Check sheet for the modelled part. Datum: model origin and axes. Units: mm. A direction names the side the tool comes from. Coordinates: 2 decimals unless noted, no trailing zeros. Loops run counter-clockwise (first coordinate to the right, second up) from the corner with the lowest first, then second, coordinate; pieces in that order, holes last. Notation, with made-up numbers: (39, 9) - (83, 9) arc R20 cw to (83, 16) - close; hole circle Ø10 at (54.25, 68). An arc over 180 degrees is marked (long way). Use a Markdown table: item, result. Add a question column.
1) Sectioned sample at D-D, the plane z = 159. Enter the section's corners in (x, y).
2) Sectioned sample at A-A, the plane y = -52. Enter the section's corners in (x, z) (1 decimal).
3) Draft check along Z on faces 6 (the flat face through (4, 1, -15.875)), 7 (the flat face through (-377, 1, 619.125)), 8 (the flat face through (3, -63.343, 0)), 9 (the cylindrical face through (-161.17, -12, 297.62)). Enter one of: pulls with the +Z half, pulls with the -Z half, needs draft (parallel to the pull), parting line crosses it, or undercut.
4) Go/stop test with flat-tipped pins: P1, Ø8, axis at x = 13.5, y = -45, coming from the +Z side (3 decimals); P2, Ø1.5, axis at y = -2, z = 51.5, coming from the -X side; P3, Ø4, axis at y = 12.5, z = 183.5, coming from the -X side. Record where each tip stops, or that it passes through.
5) Sectioned sample at B-B, the plane z = 606. Enter the section's corners in (x, y).
6) Thickness scan on line 1 (Z direction, x = -551, y = 48.5) (3 decimals); line 2 (Z direction, x = -14, y = 47.5) (3 decimals); line 3 (X direction, y = -1, z = 445). Record the ranges inside material, lowest first.
7) Tool access check on faces 1 (the cylindrical face through (-554.43, 26.93, 681.74)), 2 (the flat face through (-384, 63.657, 603)), 3 (the cylindrical face through (-253.985, -1.239, 0.222)), 4 (the cylindrical face through (-127.015, 1.554, 603.472)), 5 (the cylindrical face through (219.83, -12, -96.36)). Record the directions out of +Z, -Z, +X, -X, +Y, -Y that give a thin tool (end or side, any length) a straight path to the whole face; none if there is none.
8) Sectioned sample at C-C, the plane x = -477. Enter the section's corners in (y, z) (3 decimals).
from build123d import *

# Parameters (mm, degrees)
SKETCH1_R           = 31.75
BOSS_EXTRUDE1_DEPTH = 15.875
SKETCH2_R           = 31.75
BOSS_EXTRUDE2_DEPTH = 571.5
BOSS_EXTRUDE3_START = -190.5
SKETCH4_R           = 31.75
BOSS_EXTRUDE3_DEPTH = 190.5
BOSS_EXTRUDE4_START = 31.75
BOSS_EXTRUDE4_DEPTH = 31.75
SKETCH7_R           = 31.75
BOSS_EXTRUDE5_DEPTH = 127


with BuildPart() as part:
    # Sketch1 → Boss-Extrude1 (new, symmetric)
    with BuildSketch(Plane.XY):
        with BuildLine():
            Line((-190.5, 63.657439452), (190.5, 63.657439452))
            ThreePointArc((190.5, 63.657439452), (254, 0.157439452), (190.5, -63.342560548))
            Line((190.5, -63.342560548), (-190.5, -63.342560548))
            ThreePointArc((-190.5, -63.342560548), (-254, 0.157439452), (-190.5, 63.657439452))
        make_face()
        with Locations((190.5, 0.157439452)):
            Circle(SKETCH1_R, mode=Mode.SUBTRACT)
    extrude(amount=BOSS_EXTRUDE1_DEPTH, both=True)

    # Sketch2 → Boss-Extrude2 (add)
    with BuildSketch(Plane.XY.offset(15.875)):
        with Locations((-190.5, 0.157439452)):
            Circle(SKETCH2_R)
    extrude(amount=BOSS_EXTRUDE2_DEPTH)

    # Sketch4 → Boss-Extrude3 (add)
    with BuildSketch(Plane.XY.offset(15.875).offset(BOSS_EXTRUDE3_START)):
        with Locations((190.5, 0.157439452)):
            Circle(SKETCH4_R)
    extrude(amount=BOSS_EXTRUDE3_DEPTH)

    # Sketch6 → Boss-Extrude4 (add)
    with BuildSketch(Plane.XY.offset(587.375).offset(BOSS_EXTRUDE4_START)):
        with BuildLine():
            Line((-571.5, 63.657439452), (-190.5, 63.657439452))
            ThreePointArc((-190.5, 63.657439452), (-127, 0.157439452), (-190.5, -63.342560548))
            Line((-190.5, -63.342560548), (-571.5, -63.342560548))
            ThreePointArc((-571.5, -63.342560548), (-635, 0.157439452), (-571.5, 63.657439452))
        make_face()
    extrude(amount=-BOSS_EXTRUDE4_DEPTH)

    # Sketch7 → Boss-Extrude5 (add)
    with BuildSketch(Plane.XY.offset(619.125)):
        with Locations((-571.5, 0.157439452)):
            Circle(SKETCH7_R)
    extrude(amount=BOSS_EXTRUDE5_DEPTH)


solid = part.part
Solved:
| question | item | result |
|---|---|---|
| 1 | outline | circle Ø63.5 at (-190.5, 0.16) |
| 2 | outline | (-607.7, 587.4) - (-154.3, 587.4) - (-154.3, 619.1) - (-607.7, 619.1) - close; (-226.7, -15.9) - (226.7, -15.9) - (226.7, 15.9) - (-226.7, 15.9) - close |
| 3 | face 6 | pulls with the -Z half |
| 3 | face 7 | pulls with the +Z half |
| 3 | face 8 | needs draft |
| 3 | face 9 | undercut |
| 4 | P1 | stops at z = 15.875 |
| 4 | P2 | stops at x = -222.22 |
| 4 | P3 | stops at x = -220.52 |
| 5 | outline | (-571.5, -63.34) - (-190.5, -63.34) arc R63.5 ccw to (-190.5, 63.66) - (-571.5, 63.66) arc R63.5 ccw to start |
| 6 | line 1 | z = 587.375 to 619.125 |
| 6 | line 2 | z = -15.875 to 15.875 |
| 6 | line 3 | x = -222.23 to -158.77 |
| 7 | face 1 | +Z |
| 7 | face 2 | +Z, -Z, +X, -X, +Y |
| 7 | face 3 | -Z, -X |
| 7 | face 4 | +Z, +X |
| 7 | face 5 | -Z |
| 8 | outline | (-63.343, 587.375) - (63.657, 587.375) - (63.657, 619.125) - (-63.343, 619.125) - close |
